```python
from build123d import *

# Parameters (mm, degrees)
CROQUIS1_W               = 95
CROQUIS1_H               = 57
SALIENTE_EXTRUIR1_DEPTH  = 8
SALIENTE_EXTRUIR2_DEPTH  = 64
SALIENTE_EXTRUIR3_DEPTH  = 24
CROQUIS4_W               = 42
CROQUIS4_H               = 14
CORTAR_EXTRUIR1_DEPTH    = 8
CROQUIS5_W               = 42
CROQUIS5_H               = 7
CORTAR_EXTRUIR2_DEPTH    = 16
CORTAR_EXTRUIR3_DEPTH    = 16
SALIENTE_EXTRUIR6_DEPTH  = 8
SALIENTE_EXTRUIR8_DEPTH  = 16
SALIENTE_EXTRUIR9_DEPTH  = 40
SALIENTE_EXTRUIR10_DEPTH = 24
SALIENTE_EXTRUIR12_DEPTH = 25
CROQUIS13_W              = 49
CROQUIS13_H              = 12.5
SALIENTE_EXTRUIR13_DEPTH = 77.5
CORTAR_EXTRUIR4_DEPTH    = 19.75
CORTAR_EXTRUIR5_REACH    = 52.75


with BuildPart() as part:
    # Croquis1 → Saliente-Extruir1 (new body)
    with BuildSketch(Plane(origin=(0, 0, 0), x_dir=(1, 0, 0), z_dir=(0, 1, 0))):
        with Locations((47.5, 28.5)):
            Rectangle(CROQUIS1_W, CROQUIS1_H)
    extrude(amount=SALIENTE_EXTRUIR1_DEPTH)

    # Croquis2 → Saliente-Extruir2 (add)
    with BuildSketch(Plane(origin=(0, 8, 0), x_dir=(1, 0, 0), z_dir=(0, 1, 0))):
        Polygon((95, 0), (95, 7), (95, 53), (95, 57), (49, 57), (49, 32), (53, 33.826086957), (53, 53), (91, 53), (91, 7), (91, 0), align=None)
    extrude(amount=SALIENTE_EXTRUIR2_DEPTH)

    # Croquis3 → Saliente-Extruir3 (add)
    with BuildSketch(Plane(origin=(0, 8, 0), x_dir=(1, 0, 0), z_dir=(0, 1, 0))):
        with BuildLine():
            Line((45, 7), (91, 7))
            Line((91, 7), (91, 53))
            Line((91, 53), (53, 53))
            Line((53, 53), (53, 33.826086957))
            Line((53, 33.826086957), (49, 32))
            Line((49, 32), (24, 32))
            Line((24, 32), (24, 28))
            ThreePointArc((24, 28), (30.150757595, 13.150757595), (45, 7))
        make_face()
    extrude(amount=SALIENTE_EXTRUIR3_DEPTH)

    # Croquis4 → Cortar-Extruir1 (cut)
    with BuildSketch(Plane(origin=(0, 32, 0), x_dir=(1, 0, 0), z_dir=(0, 1, 0))):
        with BuildLine():
            ThreePointArc((38, 28), (40.050252532, 23.050252532), (45, 21))
            Line((45, 21), (45, 7))
            ThreePointArc((45, 7), (30.150757595, 13.150757595), (24, 28))
            Line((24, 28), (38, 28))
        make_face()
        with Locations((70, 14)):
            Rectangle(CROQUIS4_W, CROQUIS4_H)
    extrude(amount=-CORTAR_EXTRUIR1_DEPTH, mode=Mode.SUBTRACT)

    # Croquis5 → Cortar-Extruir2 (cut)
    with BuildSketch(Plane(origin=(0, 32, 0), x_dir=(1, 0, 0), z_dir=(0, 1, 0))):
        with BuildLine():
            ThreePointArc((45, 14), (35.100505063, 18.100505063), (31, 28))
            Line((31, 28), (24, 28))
            ThreePointArc((24, 28), (30.150757595, 13.150757595), (45, 7))
            Line((45, 7), (45, 14))
        make_face()
        with Locations((70, 10.5)):
            Rectangle(CROQUIS5_W, CROQUIS5_H)
    extrude(amount=-CORTAR_EXTRUIR2_DEPTH, mode=Mode.SUBTRACT)

    # Croquis6 → Cortar-Extruir3 (cut)
    with BuildSketch(Plane(origin=(95, 0, 0), x_dir=(0, 0, -1), z_dir=(1, 0, 0))):
        Polygon((0, 72), (0, 24), (53, 72), align=None)
    extrude(amount=-CORTAR_EXTRUIR3_DEPTH, mode=Mode.SUBTRACT)



with BuildPart() as body_2:
    # Croquis7 → Saliente-Extruir6 (new body)
    with BuildSketch(Plane(origin=(0, 32, 0), x_dir=(1, 0, 0), z_dir=(0, 1, 0))):
        Polygon((49, 32), (91, 32), (91, 39), align=None)
    extrude(amount=SALIENTE_EXTRUIR6_DEPTH)


with BuildPart() as body_3:
    # Croquis9 → Saliente-Extruir8 (new body)
    with BuildSketch(Plane(origin=(0, 32, 0), x_dir=(1, 0, 0), z_dir=(0, 1, 0))):
        Polygon((91, 39), (91, 46), (49, 32), align=None)
    extrude(amount=SALIENTE_EXTRUIR8_DEPTH)


with BuildPart() as part_1:
    add(part.part)

    add(body_2.part)  # Saliente-Extruir9 merges body 2

    add(body_3.part)  # Saliente-Extruir9 merges body 3
    # Croquis10 → Saliente-Extruir9 (add)
    with BuildSketch(Plane(origin=(0, 32, 0), x_dir=(1, 0, 0), z_dir=(0, 1, 0))):
        Polygon((49, 32), (53, 33.826086957), (53, 33.333333333), align=None)
    extrude(amount=SALIENTE_EXTRUIR9_DEPTH)

    # Croquis11 → Saliente-Extruir10 (add)
    with BuildSketch(Plane(origin=(0, 32, 0), x_dir=(1, 0, 0), z_dir=(0, 1, 0))):
        Polygon((53, 53), (53, 33.333333333), (91, 46), (91, 53), align=None)
    extrude(amount=SALIENTE_EXTRUIR10_DEPTH)

    # Croquis12 → Saliente-Extruir12 (add)
    with BuildSketch(Plane(origin=(0, 0, -32), x_dir=(-1, 0, 0), z_dir=(0, 0, -1))):
        Polygon((-49, 32), (-49, 8), (-24, 8), align=None)
    extrude(amount=SALIENTE_EXTRUIR12_DEPTH)

    # Croquis13 → Saliente-Extruir13 (add)
    with BuildSketch(Plane(origin=(0, 8, 0), x_dir=(1, 0, 0), z_dir=(0, 1, 0))):
        with Locations((24.5, 44.5)):
            Rectangle(CROQUIS13_W, CROQUIS13_H)
    extrude(amount=SALIENTE_EXTRUIR13_DEPTH)

    # Croquis14 → Cortar-Extruir4 (cut, through all)
    with BuildSketch(Plane.XY.offset(-38.25)):
        with BuildLine():
            Line((24, 32), (0, 8))
            Line((0, 8), (0, 85.5))
            Line((0, 85.5), (49, 85.5))
            Line((49, 85.5), (49, 72))
            ThreePointArc((49, 72), (36.5, 84.5), (24, 72))
            Line((24, 72), (36.5, 72))
            Line((36.5, 72), (24, 32))
        make_face()
        with BuildLine():
            Line((49, 50.75), (49, 32))
            Line((49, 32), (30.25, 32))
            ThreePointArc((30.25, 32), (35.741747853, 45.258252147), (49, 50.75))
        make_face()
    extrude(amount=-CORTAR_EXTRUIR4_DEPTH, mode=Mode.SUBTRACT)

    # Croquis15 → Cortar-Extruir5 (cut, up to next)
    with BuildSketch(Plane(origin=(0, 0, -50.75), x_dir=(-1, 0, 0), z_dir=(0, 0, -1)), mode=Mode.PRIVATE) as cortar_extruir5_sk1:
        Polygon((-30.25, 32), (-49, 32), (-30.25, 14), align=None)
    cortar_extruir5_tool1 = extrude(cortar_extruir5_sk1.sketch, amount=-CORTAR_EXTRUIR5_REACH, mode=Mode.PRIVATE) & part_1.part
    add(cortar_extruir5_tool1.solids().sort_by_distance((36.5, 26, -50.75))[0], mode=Mode.SUBTRACT)


solid = part_1.part
```
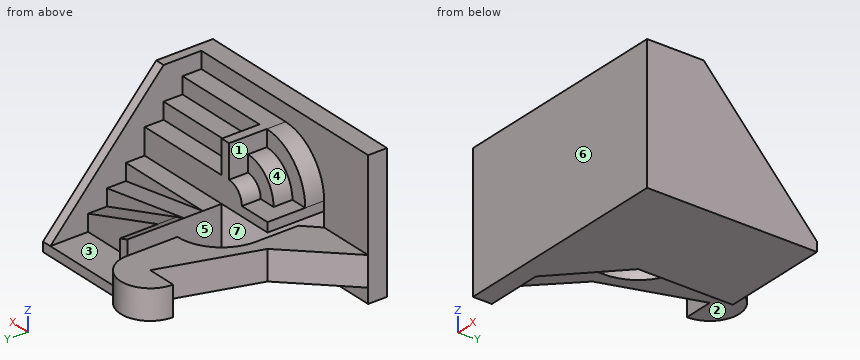
For this review, take the finished solid that the model builds, in its own axes (mm). Face numbers are marked on the shaded views. A direction names the side the tool comes from. Give positions to 0.01 mm unless a question says otherwise; leave off trailing zeros. Write each loop counter-clockwise with the first axis right and the second up, starting at its lowest first coordinate (ties: lowest second). Pieces come first, ordered by that corner, then holes. Notation, with made-up numbers: M 47,-21 L 73,-21 A21 cw 73,10 Z; hole C 79.25,-18 d9. An arc over 180 degrees is marked long. Answer as a JSON object with one key per item and string values. Group by question number.
Item 1: Draft analysis for pull direction X (two halves, no side actions). For the marked faces 4, 5, 6 and 7, state which applies: +X half, -X half, draft (parallel to the pull), parting line (faces both ways), or undercut.
Item 2: Consider section A-A on y = 20.5. Write out the cut boundary in (x, z), plus the area to 3 significant figures.
Item 3: Consider section B-B on z = -42.5. Write out the cut boundary in (x, y).
Item 4: For probe 1 along Z at (x, y) = (20, 26); probe 2 along Y at (x, z) = (57, -45.5); probe 3 along Y at (x, z) = (53.5, -6), list the stretches that pass through material, from the lowest coordinate up. Write a range as [from, to].
Item 5: Consider section C-C on x = 62.5. Write out the cut boundary in (y, z).
Item 6: Tool access review of the marked faces 1, 2 and 3: name each direction out of +Z, -Z, +X, -X, +Y, -Y from which nothing blocks a thin tool from reaching the whole face with its end or side.
Item 7: For pin 1 Ø5.5 at (x, z) = (75.5, -35.5) entering from +Y; pin 2 Ø1.5 at (y, z) = (63.5, -37.5) entering from +X; pin 3 Ø7 at (x, z) = (38.5, -21.5) entering from +Y, all flat-tipped, find the tip position at first contact; note any pin that passes through.
Item 8: Consider section D-D on z = -24.5. Write out the cut boundary in (x, y).
Check result:
{
 "1": {"face 4": "-X half", "face 5": "undercut", "face 6": "draft", "face 7": "undercut"},
 "2": {"outline": "M 12.5,-50.75 L 30.25,-50.75 L 30.25,-38.25 L 12.5,-38.25 Z; M 24,-32 L 37.02,-32 L 37.02,-57 L 95,-57 L 95,0 L 91,0 L 91,-14 L 49,-14 L 49,-7 L 45,-7 L 45,-14 A14 ccw 31,-28 L 24,-28 Z", "area": "2,890 mm^2"},
 "3": {"outline": "M 0,0 L 95,0 L 95,62.49 L 91,62.49 L 91,48 L 80.5,48 L 80.5,56 L 53,56 L 53,72 L 49,72 A12.5 ccw 24,72 L 36.5,72 L 24,32 L 0,8 Z; hole M 30.25,14 L 49,32 L 49,50.75 A18.75 ccw 30.25,32 Z"},
 "4": {"probe 1": "z = [-50.75, -38.25]", "probe 2": "y = [0, 56]", "probe 3": "y = [0, 8]"},
 "5": {"outline": "M 0,-57 L 72,-57 L 72,-53 L 56,-53 L 56,-36.5 L 48,-36.5 L 48,-34.25 L 40,-34.25 L 40,-32 L 32,-32 L 32,-21 L 24,-21 L 24,-14 L 16,-14 L 16,-7 L 8,-7 L 8,0 L 0,0 Z"},
 "6": {"face 1": "+Z, -X, +Y", "face 2": "-Z, -X, +Y", "face 3": "+Z, +Y"},
 "7": {"pin 1": "stops at y = 48", "pin 2": "stops at x = 53", "pin 3": "stops at y = 32"},
 "8": {"outline": "M 0,0 L 95,0 L 95,46.19 L 91,46.19 L 91,32 L 38.94,32 L 38.94,24 L 31.44,24 L 31.44,16 L 24.29,16 L 24.29,8 L 0,8 Z"}
}
